The listing builds one solid part. Answer for the finished solid, in the listing's coordinates (mm). A direction names the side the tool comes from. Round coordinates to 2 decimals unless told otherwise and drop trailing zeros. Write each loop counter-clockwise with the first axis right and the second up, starting at its lowest first coordinate (ties: lowest second). Pieces come first, ordered by that corner, then holes. Notation, with made-up numbers: (11, 56) - (54, 56) arc R24 cw to (54, 90) - close; hole circle Ø1 at (56, -28.5). An arc over 180 degrees is marked (long way). Answer in a Markdown table with one row per item.
from build123d import *

# Parameters (mm, degrees)
EX_BODY_DEPTH        = 210
SHELL_T              = -3
SK_FLOORHOLES_R      = 2.65
SK_FLOORHOLES_R_2    = 10
CUT_FLOORHOLES_DEPTH = 3


with BuildPart() as part:
    # SK_Body → EX_Body (new body)
    with BuildSketch(Plane(origin=(-105, 0, 0), x_dir=(0, 0, -1), z_dir=(1, 0, 0))):
        Polygon((70, 0), (-52, 0), (-52, 125), (-20, 125), (70, 61.981321561), align=None)
    extrude(amount=EX_BODY_DEPTH)

    # Shell
    shell_openings = [part.faces().sort_by_distance(p)[0] for p in [
        (0, 62.5, 52),
    ]]
    offset(amount=SHELL_T, openings=shell_openings, kind=Kind.INTERSECTION)

    # SK_FloorHoles → CUT_FloorHoles (cut)
    with BuildSketch(Plane(origin=(0, 0, 0), x_dir=(1, 0, 0), z_dir=(0, 1, 0))):
        with Locations(Location((60, 0, 0), (0, 0, 270))):
            Circle(SK_FLOORHOLES_R)
        with Locations(Location((-60, 0, 0), (0, 0, 270))):
            Circle(SK_FLOORHOLES_R)
        with Locations(Location((0, 25, 0), (0, 0, 270))):
            Circle(SK_FLOORHOLES_R_2)
    extrude(amount=CUT_FLOORHOLES_DEPTH, mode=Mode.SUBTRACT)


solid = part.part
(1) Find the intervals of material crossed by line 1 (X direction, y = 1.9, z = 0); line 2 (X direction, y = 42, z = -58.5); line 3 (X direction, y = 1.2, z = -25), in increasing order.
Checked values:
| item | result |
|---|---|
| line 1 | x = -105 to -62.65, -57.35 to 57.35, 62.65 to 105 |
| line 2 | x = -105 to -102, 102 to 105 |
| line 3 | x = -105 to -10, 10 to 105 |
(2) Section A-A (x = -60) is taken. Give the vertices of the cut face in (y, z), and give its area (3 significant figures).
Checked values:
| item | result |
|---|---|
| outline | (0, -70) - (61.98, -70) - (125, 20) - (125, 52) - (122, 52) - (122, 20.95) - (60.42, -67) - (3, -67) - (3, -2.65) - (0, -2.65) - close; (0, 2.65) - (3, 2.65) - (3, 52) - (0, 52) - close |
| area | 945 mm2 |
(3) For faces 1 (the cylindrical face through (57.649, 1.479, 1.223)), 2 (the flat face through (-1, 31, -70)), 3 (the flat face through (-1.43, 91.64, -22.41)), determine the directions among +Z, -Z, +X, -X, +Y, -Y from which every point of the face is accessible in a straight line to the end or side of a thin tool.
Checked values:
| item | result |
|---|---|
| face 1 | -Y |
| face 2 | -Z, +X, -X, +Y, -Y |
| face 3 | +Z |
(4) Section C-C (y = 27.5) is taken. Give the vertices of the cut face in (x, z), and give its area (3 significant figures).
Checked values:
| item | result |
|---|---|
| outline | (-105, -70) - (105, -70) - (105, 52) - (102, 52) - (102, -67) - (-102, -67) - (-102, 52) - (-105, 52) - close |
| area | 1,340 mm2 |
(5) Flat-ended cylindrical pins translate along their axes: pin 1 (3 mm diameter, centred on x = -18, z = -23, fed in from +Y); pin 2 (2 mm diameter, centred on x = -56.5, y = 88.5, fed in from +Z); pin 3 (6 mm diameter, centred on x = -60, z = 0, fed in from +Y). Find the tip coordinate at first contact, or state that the pin passes through.
Checked values:
| item | result |
|---|---|
| pin 1 | stops at y = 95.94 |
| pin 2 | stops at z = -25.47 |
| pin 3 | stops at y = 113.1 |
(6) Section D-D (x = 92.5) is taken. Give the vertices of the cut face in (y, z).
Checked values:
| item | result |
|---|---|
| outline | (0, -70) - (61.98, -70) - (125, 20) - (125, 52) - (122, 52) - (122, 20.95) - (60.42, -67) - (3, -67) - (3, 52) - (0, 52) - close |
(7) Section B-B (z = -6) is taken. Give the vertices of the cut face in (x, y).
Checked values:
| item | result |
|---|---|
| outline | (-105, 0) - (105, 0) - (105, 106.79) - (-105, 106.79) - close; hole (-102, 3) - (102, 3) - (102, 103.13) - (-102, 103.13) - close |
(8) For a pull along Z with two mould halves and no side action, classify faces 4 (the cylindrical face through (-62.351, 1.479, 1.223)), 5 (the flat face through (-105, 49, 4)), 6 (the flat face through (-1.47, 93.93, -24.37)), 7 (the cylindrical face through (3, 1.48, -15.46)) as pulls with the +Z half, pulls with the -Z half, needs draft (parallel to the pull), parting line crosses it, or undercut.
Checked values:
| item | result |
|---|---|
| face 4 | undercut |
| face 5 | needs draft |
| face 6 | pulls with the -Z half |
| face 7 | undercut |
